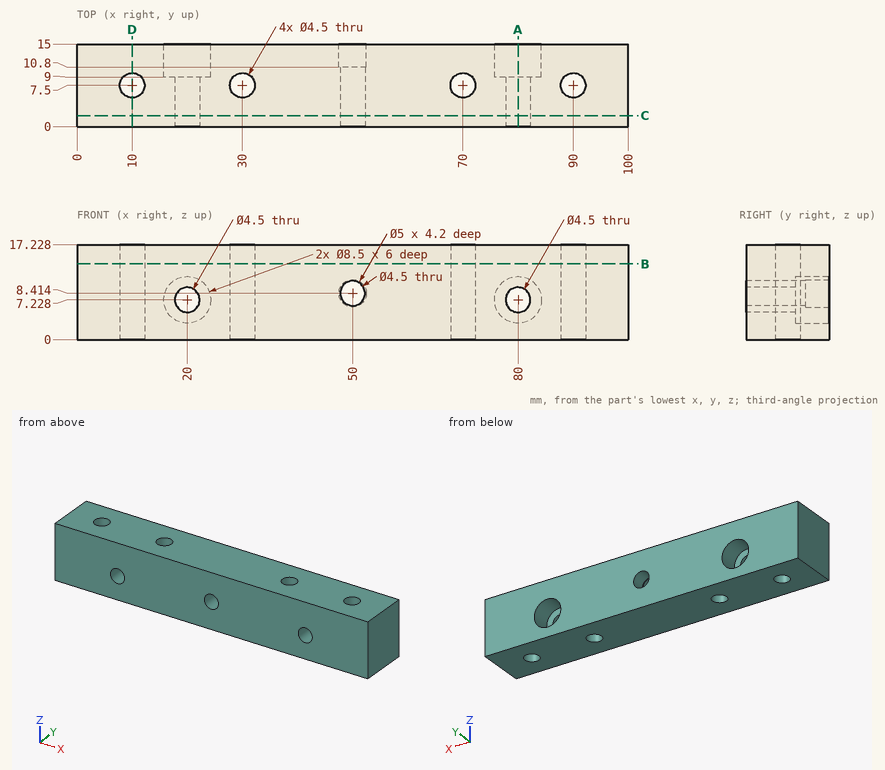
For this review, use the dimensioned drawing (mm, ordinates from the lowest corner) and the shaded views. Round coordinates to 2 decimals unless told otherwise and drop trailing zeros. Order: outer loops, then holes, each group sorted by start corner. A loop starts at its lowest first (then second) coordinate and runs counter-clockwise, first axis right, second up. Notation, with made-up numbers: (32.25, -3) - (90.25, -3) arc R24 ccw to (90.25, 14) - close; hole circle Ø4 at (62.25, 87.5). An arc over 180 degrees is marked (long way). Use one line per item in the form item = value.
Q1. Add section A-A on x = 80. Give the boundary of the cut face in (y, z), then the cut area to 3 significant figures.
Response values:
outline = (0, 0) - (15, 0) - (15, 2.98) - (9, 2.98) - (9, 4.98) - (0, 4.98) - close; (0, 9.48) - (9, 9.48) - (9, 11.48) - (15, 11.48) - (15, 17.23) - (0, 17.23) - close
area = 167 mm^2
Q2. Clearance check with a flat-ended pin moving along its axis: P1, Ø2.5, axis at x = 82, z = 6, coming from the +Y side. State where the tip first meets the part, or that it passes through.
Response values:
P1 = 9
Q3. To check wall thickness, follow line 1 (Y direction, x = 90, z = 13.5); line 2 (X direction, y = 8.75, z = 1.25); line 3 (X direction, y = 9.5, z = 14). State the ranges of each line that lie inside material, in increasing order.
Response values:
line_1 = 0 to 5.25, 9.75 to 15
line_2 = 0 to 8.13, 11.87 to 28.13, 31.87 to 68.13, 71.87 to 88.13, 91.87 to 100
line_3 = 0 to 8.97, 11.03 to 28.97, 31.03 to 68.97, 71.03 to 88.97, 91.03 to 100
Q4. Add section B-B on z = 13.75. Give the boundary of the cut face in (x, y), then the cut area to 3 significant figures.
Response values:
outline = (0, 0) - (100, 0) - (100, 15) - (0, 15) - close; hole circle Ø4.5 at (10, 7.5); hole circle Ø4.5 at (30, 7.5); hole circle Ø4.5 at (70, 7.5); hole circle Ø4.5 at (90, 7.5)
area = 1,440 mm^2
Q5. Add section D-D on x = 10. Give the boundary of the cut face in (y, z), then the cut area to 3 significant figures.
Response values:
outline = (0, 0) - (5.25, 0) - (5.25, 17.23) - (0, 17.23) - close; (9.75, 0) - (15, 0) - (15, 17.23) - (9.75, 17.23) - close
area = 181 mm^2
Q6. Add section C-C on y = 2. Give the boundary of the cut face in (x, z).
Response values:
outline = (0, 0) - (100, 0) - (100, 17.23) - (0, 17.23) - close; hole circle Ø4.5 at (20, 7.23); hole circle Ø4.5 at (50, 8.41); hole circle Ø4.5 at (80, 7.23)
